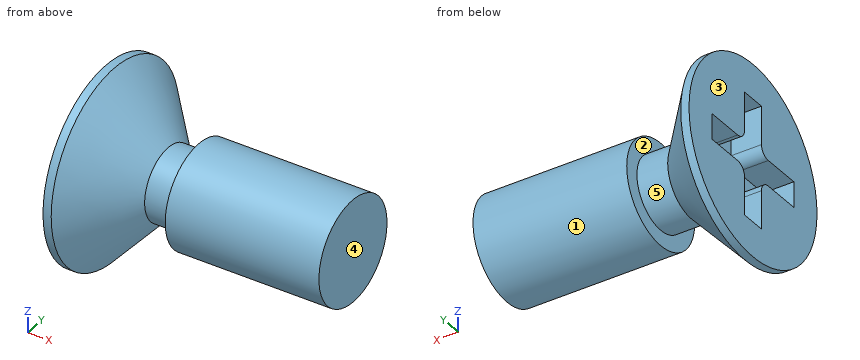
```python
from build123d import *

# Parameters (mm, degrees)
CUT_EXTRUDE_1_DEPTH = 0.75


with BuildPart() as part:
    # 草图1 → 旋转1 (revolve)
    with BuildSketch(Plane.XY):
        Polygon((0, 0), (0, 1.25), (-3.75, 1.25), (-3.75, 0.875), (-4.5, 0.875), (-5.8, 2.35), (-6, 2.35), (-6, 0), align=None)
    revolve(axis=Axis((0, 0, 0), (-1, 0, 0)))

    # 草图2 → 切除-拉伸1 (cut)
    with BuildSketch(Plane.ZY.offset(6)):
        with BuildLine():
            Line((-0.3125, 1.5), (0.3125, 1.5))
            Line((0.3125, 1.5), (0.3125, 0.5625))
            ThreePointArc((0.3125, 0.5625), (0.385723305, 0.385723305), (0.5625, 0.3125))
            Line((0.5625, 0.3125), (1.5, 0.3125))
            Line((1.5, 0.3125), (1.5, -0.3125))
            Line((1.5, -0.3125), (0.5625, -0.3125))
            ThreePointArc((0.5625, -0.3125), (0.385723305, -0.385723305), (0.3125, -0.5625))
            Line((0.3125, -0.5625), (0.3125, -1.5))
            Line((0.3125, -1.5), (-0.3125, -1.5))
            Line((-0.3125, -1.5), (-0.3125, -0.5625))
            ThreePointArc((-0.3125, -0.5625), (-0.385723305, -0.385723305), (-0.5625, -0.3125))
            Line((-0.5625, -0.3125), (-1.5, -0.3125))
            Line((-1.5, -0.3125), (-1.5, 0.3125))
            Line((-1.5, 0.3125), (-0.5625, 0.3125))
            ThreePointArc((-0.5625, 0.3125), (-0.385723305, 0.385723305), (-0.3125, 0.5625))
            Line((-0.3125, 0.5625), (-0.3125, 1.5))
        make_face()
    extrude(amount=-CUT_EXTRUDE_1_DEPTH, mode=Mode.SUBTRACT)


solid = part.part
```
Could you check a few things on this model? Use its own coordinates, in mm. Face numbers are marked on the shaded views. A direction names the side the tool comes from. Coordinates: 2 decimals unless noted, no trailing zeros. Loops run counter-clockwise (first coordinate to the right, second up) from the corner with the lowest first, then second, coordinate; pieces in that order, holes last.
1) Imagine slicing it at C-C (x = -3.65). List the corners of the cut face in (y, z) for me, and give its area (3 significant figures).
Reported:
outline: circle Ø2.5 at (0, 0)
area: 4.91 mm2
2) Please list where these lines run through material, in increasing order: line 1 along X through (y, z) = (0.4, -0.1); line 2 along Z through (x, y) = (-2.7, -0.05); line 3 along Z through (x, y) = (-5.75, 0.4).
Reported:
line 1: x = -5.25 to 0
line 2: z = -1.25 to 1.25
line 3: z = -2.26 to -0.37, 0.37 to 2.26
3) Imagine slicing it at A-A (y = 0). List the corners of the cut face in (x, z) for me (3 decimals), and give its area (3 significant figures).
Reported:
outline: (-6, -2.35) - (-5.8, -2.35) - (-4.5, -0.875) - (-3.75, -0.875) - (-3.75, -1.25) - (0, -1.25) - (0, 1.25) - (-3.75, 1.25) - (-3.75, 0.875) - (-4.5, 0.875) - (-5.8, 2.35) - (-6, 2.35) - (-6, 1.5) - (-5.25, 1.5) - (-5.25, -1.5) - (-6, -1.5) - close
area: 13.6 mm2
4) Will these pins go through, and if not, where does the flat tip stop? pin 1 Ø0.6 at (x, y) = (-6, -1) entering from -Z; pin 2 Ø0.6 at (x, z) = (-5.5, -1) entering from -Y; pin 3 Ø1 at (x, z) = (-3.5, -0.5) entering from -Y.
Reported:
pin 1: stops at z = -2.24
pin 2: stops at y = -2.15
pin 3: stops at y = -1.25
5) Thinking about a two-plate mould opening in X: for the marked faces 1, 2 and 3, which applies, released by +X, released by -X, zero draft, split by the parting line, or undercut?
Reported:
face 1: zero draft
face 2: undercut
face 3: released by -X
6) Which directions (+Z, -Z, +X, -X, +Y, -Y) give clear straight access to the entire face, cutting with the end or side of a thin tool? Please do the marked faces 4 and 5.
Reported:
face 4: +Z, -Z, +X, +Y, -Y
face 5: none
